Here's how the part is built. I have some questions about the finished solid (model axes, mm). Face numbers are marked on the shaded views. A direction names the side the tool comes from. Give positions to 0.01 mm unless a question says otherwise; leave off trailing zeros. Loops run counter-clockwise (first coordinate to the right, second up) from the corner with the lowest first, then second, coordinate; pieces in that order, holes last.
Q1. I need wall thicknesses on probe 1 along Y at (x, z) = (-39, -0.5); probe 2 along Y at (x, z) = (-19, 2.25); probe 3 along Z at (x, y) = (30.5, 4). Which ranges of each line are inside material? Lowest first, please.
Q2. Suppose I cut it at B-B (x = -33). List the corners of the cut face in (y, z) for me, and give its area (3 significant figures).
Q3. I'm going to push flat-ended pins straight in: P1, Ø5, axis at x = 26, z = 3.5, coming from the -Y side; P2, Ø6, axis at x = 27.5, z = 6, coming from the -Y side; P3, Ø8, axis at x = 12.5, y = 5, coming from the +Z side (3 decimals); P4, Ø4, axis at x = -21, y = 0.5, coming from the +Z side. Where does each tip first touch, or does it pass through?
Q4. Suppose I cut it at A-A (x = -1). List the corners of the cut face in (y, z) for me (3 decimals).
Q5. For the marked faces 1, 2 and 3, which set-ups out of +Z, -Z, +X, -X, +Y, -Y let a thin tool reach every point of the face, with its end or its side?
```python
from build123d import *

# Parameters (mm, degrees)
F1_DEPTH = 13.081
F2_R     = 9.398
F3_DEPTH = 36.576
F4_SIZE  = 1.524


with BuildPart() as f1:
    # F0 (on Right) → F1 (new body)
    with BuildSketch(Plane.YZ):
        Polygon((5.499261, -9.525), (10.998523, 0), (5.499261, 9.525), (-5.499261, 9.525), (-10.998523, 0), (-5.499261, -9.525), align=None)
    extrude(amount=F1_DEPTH)

    # F2 (on face) → F3 (join)
    with BuildSketch(Plane.YZ.offset(13.081)):
        Circle(F2_R)
    extrude(amount=F3_DEPTH)

    # F4
    f4_edges = [f1.edges().sort_by_distance(p)[0] for p in [
        (49.657, -9.398, 0),
    ]]
    chamfer(f4_edges, length=F4_SIZE)

    # F5 (on Top) → F6 (revolve, cut)
    with BuildSketch(Plane.XY):
        Polygon((13.081, 9.398), (13.081, 11.43), (11.049, 11.43), align=None)
    revolve(axis=Axis((19.661747, 0, 0), (-1, 0, 0)), mode=Mode.SUBTRACT)

    # F7: F1 across face


with BuildPart() as f1_1:
    add(f1.part)
    add(f1.part.mirror(Plane(origin=(0, 0, 0), x_dir=(0, 1, 0), z_dir=(-1, 0, 0))))


solid = f1_1.part
```
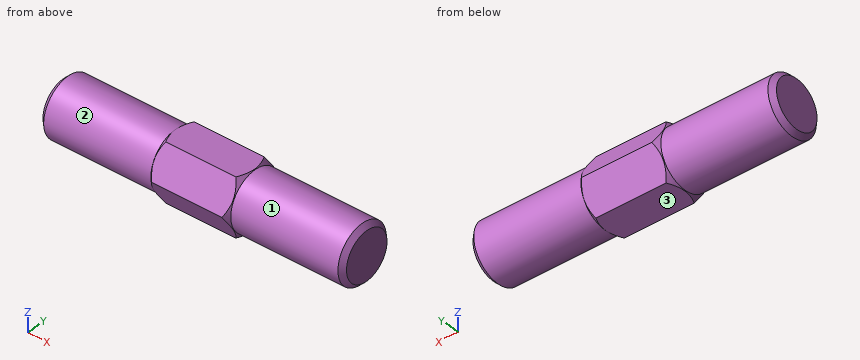
Solutions:
1. probe 1: y = -9.38 to 9.38
1. probe 2: y = -9.12 to 9.12
1. probe 3: z = -8.5 to 8.5
2. outline: circle Ø18.8 at (0, 0)
2. area: 277 mm2
3. P1: stops at y = -9.34
3. P2: stops at y = -8.91
3. P3: stops at z = 9.525
3. P4: stops at z = 9.4
4. outline: (-10.999, 0) - (-5.499, -9.525) - (5.499, -9.525) - (10.999, 0) - (5.499, 9.525) - (-5.499, 9.525) - close
5. face 1: +X
5. face 2: -X
5. face 3: -Z, +X, -X, +Y, -Y
